Can you work these out from the drawing? Everything is in mm from the part's minimum corner. A direction names the side the tool comes from. Coordinates: 2 decimals unless noted, no trailing zeros. Write each loop counter-clockwise with the first axis right and the second up, starting at its lowest first coordinate (ties: lowest second). Pieces come first, ordered by that corner, then holes. Notation, with made-up numbers: (27.25, -16.75) -> (60.25, -16.75) arc R24 ccw to (60.25, 2.25) -> close; hole circle Ø1 at (23, -39.75). An arc over 180 degrees is marked (long way). Use a Markdown table: item, result. Add a question column.
Item 1: If we mould it in two halves opening along Y, with no side actions, what happens to the marked faces 3, 4 and 5? For each: pulls with the +Y half, pulls with the -Y half, needs draft (parallel to the pull), parting line crosses it, or undercut.
Item 2: On a 3-axis mill with a long thin cutter (end or side, diameter ignored), from which of +Z, -Z, +X, -X, +Y, -Y can I reach the whole of each face in a straight line? I mean the marked faces 1 and 2. Say none if no direction works.
Item 3: Imagine slicing it at A-A, the plane y = 9. Write out the boundary of the cut face in (x, z).
Item 4: Will these pins go through, and if not, where does the flat tip stop? pin 1 Ø4.5 at (y, z) = (9, 22) entering from -X; pin 2 Ø5.5 at (x, y) = (26.5, 12.5) entering from +Z.
Item 5: If I drill on line 1 along X through (y, z) = (2.5, 10); line 2 along Z through (x, y) = (38.5, 9); line 3 along Y through (x, z) = (30, 2), over which ranges is the centre line in solid material (lowest first)? Write a range as from..to.
Item 6: Imagine slicing it at C-C, the plane x = 30. Write out the boundary of the cut face in (y, z).
Item 7: Imagine slicing it at D-D, the plane y = 5.5. Write out the boundary of the cut face in (x, z), and give its area (3 significant figures).
Item 8: Imagine slicing it at B-B, the plane z = 22. Write out the boundary of the cut face in (x, y).
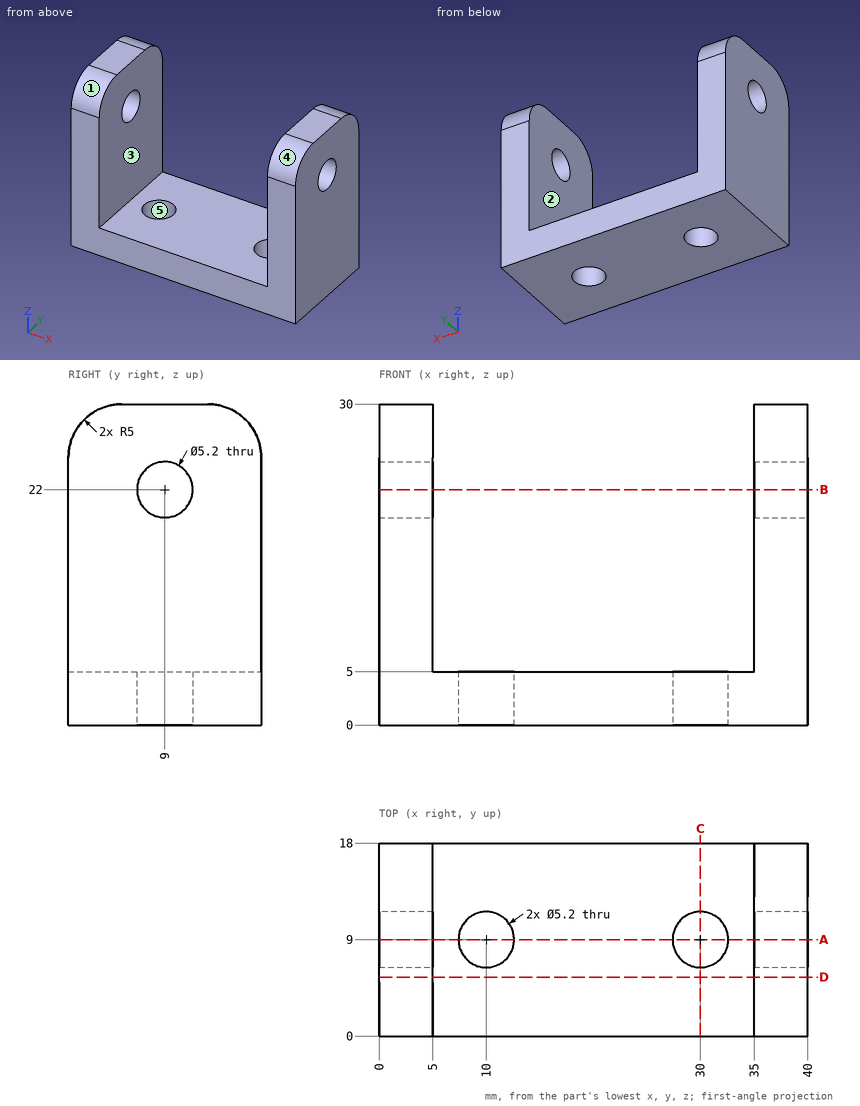
Ans:
| question | item | result |
|---|---|---|
| 1 | face 3 | needs draft |
| 1 | face 4 | pulls with the -Y half |
| 1 | face 5 | undercut |
| 2 | face 1 | +Z, +X, -X, -Y |
| 2 | face 2 | +Z, +Y, -Y |
| 3 | outline | (0, 0) -> (7.4, 0) -> (7.4, 5) -> (5, 5) -> (5, 19.4) -> (0, 19.4) -> close; (0, 24.6) -> (5, 24.6) -> (5, 30) -> (0, 30) -> close; (12.6, 0) -> (27.4, 0) -> (27.4, 5) -> (12.6, 5) -> close; (32.6, 0) -> (40, 0) -> (40, 19.4) -> (35, 19.4) -> (35, 5) -> (32.6, 5) -> close; (35, 24.6) -> (40, 24.6) -> (40, 30) -> (35, 30) -> close |
| 4 | pin 1 | passes through |
| 4 | pin 2 | stops at z = 5 |
| 5 | line 1 | x = 0..5, 35..40 |
| 5 | line 2 | z = 0..19.4, 24.6..30 |
| 5 | line 3 | y = 0..6.4, 11.6..18 |
| 6 | outline | (0, 0) -> (6.4, 0) -> (6.4, 5) -> (0, 5) -> close; (11.6, 0) -> (18, 0) -> (18, 5) -> (11.6, 5) -> close |
| 7 | outline | (0, 0) -> (40, 0) -> (40, 30) -> (35, 30) -> (35, 5) -> (5, 5) -> (5, 30) -> (0, 30) -> close |
| 7 | area | 450 mm^2 |
| 8 | outline | (0, 0) -> (5, 0) -> (5, 6.4) -> (0, 6.4) -> close; (0, 11.6) -> (5, 11.6) -> (5, 18) -> (0, 18) -> close; (35, 0) -> (40, 0) -> (40, 6.4) -> (35, 6.4) -> close; (35, 11.6) -> (40, 11.6) -> (40, 18) -> (35, 18) -> close |
